```python
from build123d import *

# Parameters (mm, degrees)
F0_W     = 156.972
F0_H     = 19.0483668515
F1_W     = 20.828
F1_H     = 19.0483668515
F3_ANGLE = 180
F4_ANGLE = 90
F5_R     = 9.525
F6_DEPTH = 20.828
F7_SIZE2 = 1.524
F7_SIZE  = 1.524


with BuildPart() as f2:
    # F0 (on Front) → F2 (revolve)
    with BuildSketch(Plane.XZ):
        with Locations((0, 9.5241834258)):
            Rectangle(F0_W, F0_H)
    revolve(axis=Axis((0, 0, 0), (-1, 0, 0)))

    # F1 (on Front) → F3 (revolve)
    with BuildSketch(Plane.XZ):
        with Locations((88.9, 9.5241834258)):
            Rectangle(F1_W, F1_H)
    revolve(axis=Axis((88.9, 0, 0), (1, 0, 0)), revolution_arc=F3_ANGLE)

    # F3_face (on face) → F4 (revolve)
    with BuildSketch(Plane(origin=(99.314, -8.0843779793, 0), x_dir=(0, 1, 0), z_dir=(1, 0, 0))):
        with BuildLine():
            ThreePointArc((8.0843779793, 19.0483668515), (-10.9639888722, 0), (8.0843779793, -19.0483668515))
            Line((8.0843779793, -19.0483668515), (8.0843779793, 19.0483668515))
        make_face()
    revolve(axis=Axis((99.314, 0, 0), (0, 0, 1)), revolution_arc=F4_ANGLE)

    # F5 (on Front) → F6 (join)
    with BuildSketch(Plane.XZ):
        with Locations((99.314, 0)):
            Circle(F5_R)
    extrude(amount=-F6_DEPTH)

    # F7
    f7_edges = [f2.edges().sort_by_distance(p)[0] for p in [
        (89.789, 20.828, 0),
    ]]
    chamfer(f7_edges, length=F7_SIZE, length2=F7_SIZE2)


solid = f2.part
```
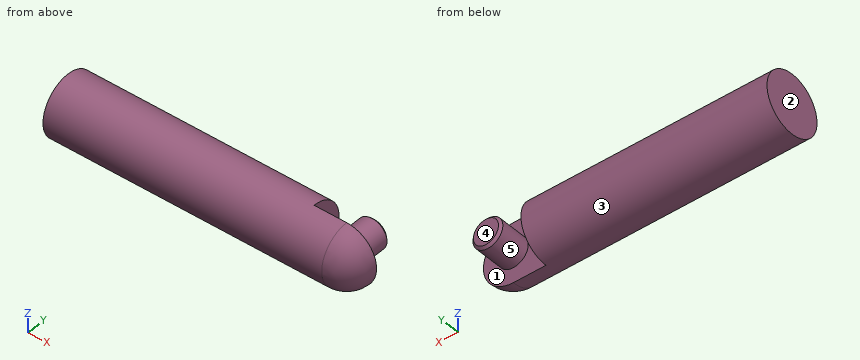
Can you work these out from the model? Positions are in its coordinate system, mm. Face numbers are marked on the shaded views. A direction names the side the tool comes from. Coordinates: 2 decimals unless noted, no trailing zeros. Loops run counter-clockwise (first coordinate to the right, second up) from the corner with the lowest first, then second, coordinate; pieces in that order, holes last.
Item 1: Which directions (+Z, -Z, +X, -X, +Y, -Y) give clear straight access to the entire face, cutting with the end or side of a thin tool? Please do the marked faces 4 and 5.
Answers below:
face 4: +Z, -Z, +X, -X, +Y
face 5: +Y
Item 2: I'm going to push flat-ended pins straight in: pin 1 (2 mm diameter, centred on y = 15, z = 3, fed in from +X); pin 2 (5 mm diameter, centred on x = 20.5, y = 7.5, fed in from -Z); pin 3 (4 mm diameter, centred on x = -12.5, y = 5.5, fed in from +Z). Where does each tip first touch, or does it pass through?
Answers below:
pin 1: stops at x = 108.63
pin 2: stops at z = -18.38
pin 3: stops at z = 18.72
Item 3: Suppose I cut it at B-B (y = 4.5). Please give me the cut outline in (x, z) (3 decimals).
Answers below:
outline: (-78.486, -18.509) - (78.486, -18.509) - (78.486, 18.509) - (-78.486, 18.509) - close; circle Ø19.05 at (99.314, 0)
Item 4: Suppose I cut it at D-D (y = -4). Please give me the cut outline in (x, z).
Answers below:
outline: (-78.49, -18.62) - (99.31, -18.62) arc R18.62 ccw to (99.31, 18.62) - (-78.49, 18.62) - close
Item 5: Please list where these lines run through material, in increasing order: L1, parallel to Z at x = 94, y = -1; L2, parallel to Y at x = 11, z = 0; L3, parallel to X at y = 2.5, z = 11.5.
Answers below:
L1: z = -19.02 to 19.02
L2: y = -19.05 to 19.05
L3: x = -78.49 to 78.49
Item 6: Suppose I cut it at A-A (z = 0). Please give me the cut outline in (x, y) (3 decimals).
Answers below:
outline: (-78.486, -19.048) - (99.314, -19.048) arc R19.048 ccw to (118.362, 0) - (108.839, 0) - (108.839, 19.304) - (107.315, 20.828) - (91.313, 20.828) - (89.789, 19.304) - (89.789, 0) - (78.486, 0) - (78.486, 19.048) - (-78.486, 19.048) - close
Item 7: If we mould it in two halves opening along X, with no side actions, what happens to the marked faces 1, 2 and 3? For each: released by +X, released by -X, zero draft, split by the parting line, or undercut.
Answers below:
face 1: undercut
face 2: released by -X
face 3: zero draft
Item 8: Suppose I cut it at C-C (x = 82). Please give me the cut outline in (y, z).
Answers below:
outline: (0, -19.05) - (0, 19.05) arc R19.05 ccw to start
